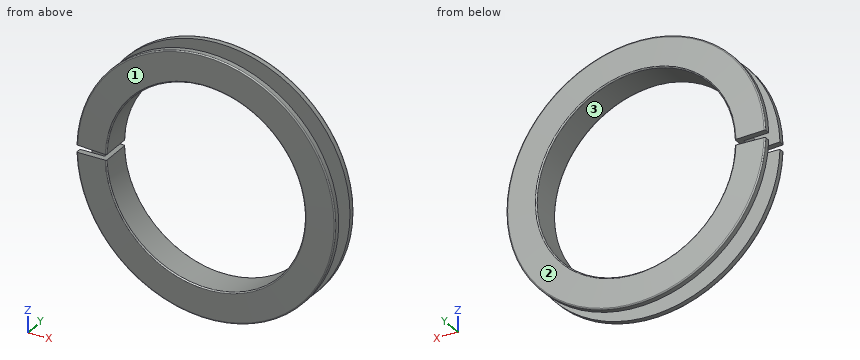
from build123d import *


with BuildPart() as part:
    # ｽｲｰﾌﾟ1: sweep along a path in ｽｹｯﾁ2
    with BuildLine(Plane(origin=(0, 0, 0), x_dir=(1, 0, 0), z_dir=(0, 1, 0))) as sweep_1_path:
        ThreePointArc((-35.993054215, -0.5), (0, 0), (-35.993054215, 0.5))
    # ｽｹｯﾁ1 → ｽｲｰﾌﾟ1 (sweep)
    with BuildSketch(Plane.XY):
        with BuildLine():
            Line((4.3, -1.6), (4.3, -2.391846945))
            ThreePointArc((4.3, -2.391846945), (4.242241142, -2.532443736), (4.102325424, -2.591833425))
            Line((4.102325424, -2.591833425), (-0.697674576, -2.647647379))
            ThreePointArc((-0.697674576, -2.647647379), (-0.840596791, -2.58990204), (-0.9, -2.447660898))
            Line((-0.9, -2.447660898), (-0.9, 2.447660898))
            ThreePointArc((-0.9, 2.447660898), (-0.840596791, 2.58990204), (-0.697674576, 2.647647379))
            Line((-0.697674576, 2.647647379), (4.102325424, 2.591833425))
            ThreePointArc((4.102325424, 2.591833425), (4.242241142, 2.532443736), (4.3, 2.391846945))
            Line((4.3, 2.391846945), (4.3, 1.6))
            Line((4.3, 1.6), (0, 1.65))
            Line((0, 1.65), (0, -1.65))
            Line((0, -1.65), (4.3, -1.6))
        make_face()
    sweep(path=sweep_1_path.line)


solid = part.part
Geometry check sheet. Reference: the model listing, model coordinates, mm. Face numbers are marked on the shaded views. A direction names the side the tool comes from. Coordinates: 2 decimals unless noted, no trailing zeros. Order: outer loops, then holes, each group sorted by start corner. A loop starts at its lowest first (then second) coordinate and runs counter-clockwise, first axis right, second up. Notation, with made-up numbers: (-2.75, -32.5) -> (32.25, -32.5) arc R28 cw to (32.25, -7.5) -> close; hole circle Ø5 at (-29.5, 53). An arc over 180 degrees is marked (long way). Use a Markdown table: item, result. Add a question column.
1. Go/stop test with flat-tipped pins: pin 1 Ø3 at (y, z) = (-2, 3) entering from +X; pin 2 Ø1 at (x, y) = (-27.5, 1.5) entering from -Z; pin 3 Ø2 at (y, z) = (1.5, -15.5) entering from +X. Record where each tip stops, or that it passes through.
2. Set-up check for the marked faces 1, 2 and 3: record each of +Z, -Z, +X, -X, +Y, -Y from which the full face is reachable in a straight line by a thin tool's end or side.
3. Cross-section at A-A (x = -37). Give the number of separate pieces and of enclosed holes in the cut face, and give its area (3 significant figures).
4. Material ranges on L1, parallel to Z at x = -18, y = -0.35; L2, parallel to Y at x = -2.5, z = 8.5; L3, parallel to Z at x = -30, y = 1.45, recorded low to high.
5. Cross-section at B-B (y = 0.45). Enter the section's corners in (x, z) (3 decimals).
Filled sheet:
| question | item | result |
|---|---|---|
| 1 | pin 1 | x = 4.25 |
| 1 | pin 2 | z = -20.4 |
| 1 | pin 3 | x = -1.06 |
| 2 | face 1 | -Y |
| 2 | face 2 | +Y |
| 2 | face 3 | +Y, -Y |
| 3 | separate pieces | 4 |
| 3 | enclosed holes | 0 |
| 3 | area | 44.1 mm2 |
| 4 | L1 | -18 to -17.1, 17.1 to 18 |
| 4 | L2 | -2.64 to 2.64 |
| 4 | L3 | -13.42 to -12.18, 12.18 to 13.42 |
| 5 | outline | (-35.993, -0.5) arc R18 ccw (long way) to (-35.993, 0.5) -> (-35.093, 0.475) arc R17.1 cw (long way) to (-35.093, -0.475) -> close |
